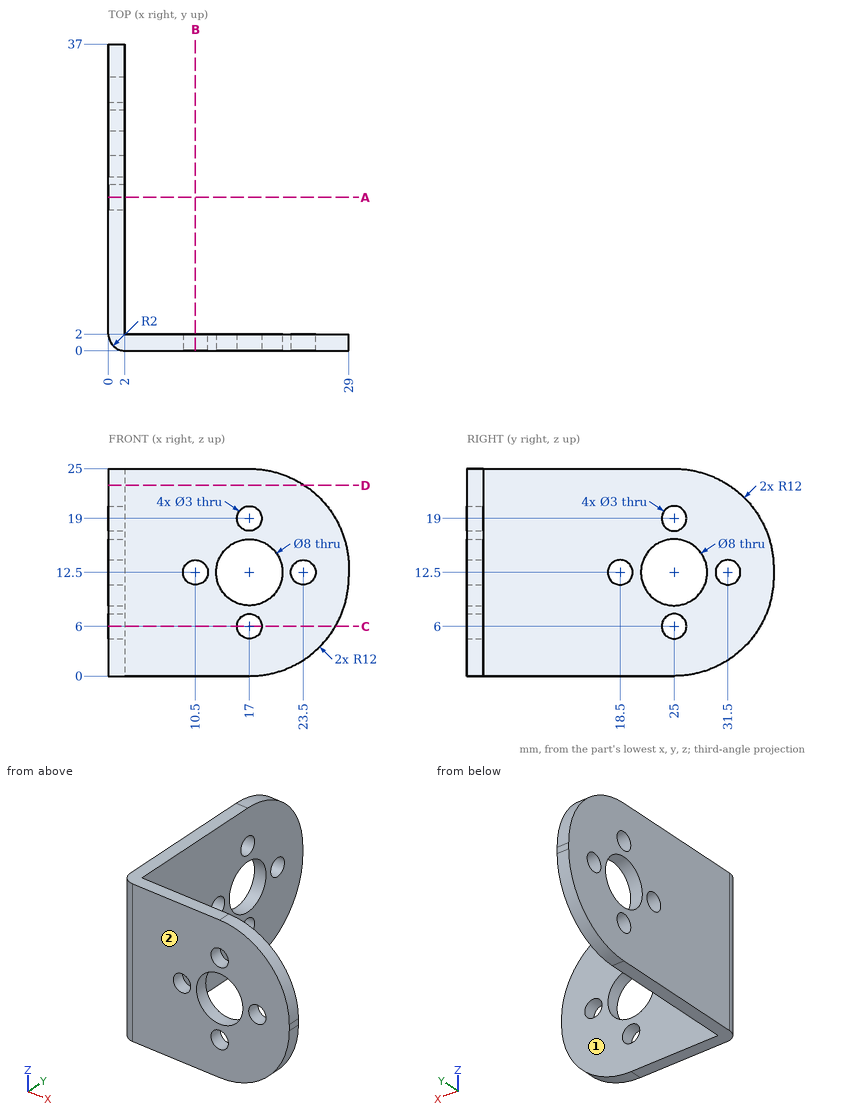
Design review of the part shown in the three views and the two pictorial views. Dimensions are in mm from the part's minimum x, y and z. A direction names the side the tool comes from. Give positions to 0.01 mm unless a question says otherwise; leave off trailing zeros. Loops run counter-clockwise (first coordinate to the right, second up) from the corner with the lowest first, then second, coordinate; pieces in that order, holes last. Notation, with made-up numbers: (81, -7.75) -> (87, -7.75) arc R16 cw to (87, 8.25) -> close; hole circle Ø3 at (14, -11.75). An arc over 180 degrees is marked (long way). Put each result on its own line as item: value. Start each with the question number.
1. We need section A-A on y = 18.5. State the section outline as (x, z) points, then the cut area to 3 significant figures.
2. We need section D-D on z = 23. State the section outline as (x, y) points, then the cut area to 3 significant figures.
3. Clearance check with flat-ended pins moving along their axes: P1, Ø6, axis at y = 15, z = 15, coming from the +X side; P2, Ø10.5, axis at x = 17, z = 12.5, coming from the +Y side; P3, Ø8, axis at x = 4.5, y = 29, coming from the +Z side. State where each tip first meets the part, or that it passes through.
4. For the marked faces 1 and 2, list the 3-axis set-ups (+Z, -Z, +X, -X, +Y, -Y) from which the entire face can be reached by the end or side of a thin tool; tool diameter is ignored.
5. We need section C-C on z = 6. State the section outline as (x, y) points, then the cut area to 3 significant figures.
6. Wall thickness on probe 1 along Z at (x, y) = (17, 1.25); probe 2 along Z at (x, y) = (0.8, 18.5); probe 3 along X at (y, z) = (19.5, 16.75): over which ranges is each line inside the solid? List them lowest first.
Determined:
1. outline: (0, 0) -> (2, 0) -> (2, 11) -> (0, 11) -> close; (0, 14) -> (2, 14) -> (2, 25) -> (0, 25) -> close
1. area: 44.0 mm^2
2. outline: (0, 2) arc R2 ccw to (2, 0) -> (23.63, 0) -> (23.63, 2) -> (2, 2) -> (2, 31.63) -> (0, 31.63) -> close
2. area: 106 mm^2
3. P1: x = 2
3. P2: y = 2
3. P3: z = 24.97
4. face 1: +Z, -Z, +X, +Y
4. face 2: +Z, -Z, +X, -X, -Y
5. outline: (0, 2) arc R2 ccw to (2, 0) -> (15.5, 0) -> (15.5, 2) -> (2, 2) -> (2, 23.5) -> (0, 23.5) -> close; (0, 26.5) -> (2, 26.5) -> (2, 35.39) -> (0, 35.39) -> close; (18.5, 0) -> (27.39, 0) -> (27.39, 2) -> (18.5, 2) -> close
5. area: 109 mm^2
6. probe 1: 0 to 4.5, 7.5 to 8.5, 16.5 to 17.5, 20.5 to 25
6. probe 2: 0 to 11, 14 to 25
6. probe 3: 0 to 2
